Build history of the part. All positions in model axes, mm. Round coordinates to 2 decimals unless told otherwise and drop trailing zeros. Loops run counter-clockwise (first coordinate to the right, second up) from the corner with the lowest first, then second, coordinate; pieces in that order, holes last. Notation, with made-up numbers: (61, 48.25) - (78, 48.25) arc R14 ccw to (78, 70.25) - close; hole circle Ø2 at (75.25, 65.25). An arc over 180 degrees is marked (long way). Use a Markdown table: item, result.
Autodesk Inventor part; units mm, degrees
ref_plane "YZ Plane" through (0, 0, 0) normal (1, 0, 0) x (0, 1, 0)
ref_plane "XZ Plane" through (0, 0, 0) normal (0, 1, 0) x (-1, 0, 0)
ref_plane "XY Plane" through (0, 0, 0) normal (0, 0, 1) x (1, 0, 0)
sketch "Sketch1" plane through (0, 0, 0) normal (0, 0, 1) x (1, 0, 0)
  line L0 (-49.2977, 34.5359) -> (-22.38, 61.3045)
  line L1 (-47.8874, 33.1177) -> (-20.9698, 59.8864)
  line L2 (-49.2977, 34.5359) -> (-47.8874, 33.1177) construction
  circle A0 centre (-52.4729, 29.968) radius 5.563
  circle A1 centre (-52.4729, 29.968) radius 3.9984
  circle A2 centre (-17.7815, 64.4351) radius 5.563
  circle A3 centre (-17.7815, 64.4351) radius 3.9984
  line L3 (-13.9364, 68.4553) -> (0.7038, 78.9274)
  line L4 (-12.7631, 66.8356) -> (1.8771, 77.3077)
  line L5 (-57.711, 28.0946) -> (-68.2683, 22.3899)
  line L6 (-56.7093, 26.3625) -> (-67.2666, 20.6578)
  line L7 (-49.5894, 25.2106) -> (10.1162, -41.4966)
  circle A4 centre (14.4958, -44.9268) radius 5.563
  circle A5 centre (14.4958, -44.9268) radius 3.9984
  circle A6 centre (52.6405, -7.8239) radius 3.9984
  circle A7 centre (52.6405, -7.8239) radius 5.563
  line L8 (-48.0932, 26.5378) -> (11.6124, -40.1694)
  line L9 (-14.6001, 59.8716) -> (48.0505, -4.6808)
  line L10 (-13.1915, 61.292) -> (49.4591, -3.2604)
  line L11 (49.4227, -12.3618) -> (19.1106, -41.8201)
  line L12 (48.0258, -10.9306) -> (17.7136, -40.3888)
  line L13 (11.2885, -49.4721) -> (3.1929, -57.3557)
  line L14 (9.8883, -48.0441) -> (1.7927, -55.9277)
  line L15 (57.2511, -4.7111) -> (65.8331, 3.6764)
  line L16 (55.8523, -3.2817) -> (64.4343, 5.1058)
  line L17 (-39.0119, 41.9442) -> (29.6903, -28.7495)
  line L18 (-37.5936, 43.3546) -> (31.1246, -27.3556)
  line L19 (-55.5021, 34.6339) -> (-63.8979, 55.9393)
  line L20 (-53.6558, 35.4038) -> (-62.0516, 56.7092)
  line L21 (-23.223, 65.5915) -> (-56.073, 66.1322)
  line L22 (-23.2803, 63.5921) -> (-56.1303, 64.1329)
  circle A8 centre (-17.2221, 20.9576) radius 3.1804
  line L23 (13.0651, -39.5509) -> (-14.9644, 18.7175)
  line L24 (11.2563, -40.4044) -> (-16.7485, 17.8127)
  line L25 (-14.0533, 20.686) -> (47.9022, -4.9092)
  line L26 (-14.8421, 18.848) -> (47.1775, -6.7738)
  line L27 (-18.703, 58.9489) -> (-18.2564, 23.9652)
  line L28 (-16.7032, 58.9776) -> (-16.2565, 23.9879)
  line L29 (-47.4654, 27.5447) -> (-20.389, 20.6653)
  line L30 (-46.932, 29.4728) -> (-19.9371, 22.614)
  line L31 (0.7038, 78.9274) -> (1.8771, 77.3077)
  line L32 (-56.073, 66.1322) -> (-56.1303, 64.1329)
  line L33 (-62.0516, 56.7092) -> (-63.8979, 55.9393)
  line L34 (-68.2683, 22.3899) -> (-67.2666, 20.6578)
  line L35 (3.1929, -57.3557) -> (1.7927, -55.9277)
  line L36 (65.8331, 3.6764) -> (64.4343, 5.1058)
  point P0 (0, 0)
  point P1 (9.143, -43.4122)
  point P2 (-19.963, 60.8956)
  point P3 (18.6755, -41.2556)
  point P4 (19.8991, -43.603)
  point P5 (47.2964, -9.3692)
  point P6 (58.0343, -9.1855)
  point P7 (55.8444, -3.2761)
  point P8 (16.2732, -50.1982)
  point P9 (18.0227, -49.2289)
  point P10 (56.2951, -12.0181)
  point P11 (57.5423, -10.4544)
  point P12 (-20.321, 22.7115)
  point P13 (-20.9757, 59.8805)
  point P14 (-18.6091, 23.8197)
  point P15 (10.5981, -39.0362)
  point P16 (31.0842, -30.1838)
  point P17 (32.5185, -28.7899)
  point P18 (31.1246, -27.3556)
  point P19 (-13.0632, 18.1131)
  point P20 (-13.5186, 15.7119)
  point P21 (29.6903, -28.7495)
  point P22 (-20.0433, 22.4258)
  dimension "d49" = 6.3609
  dimension "d0" = 2
  dimension "d2" = 1
  dimension "d3" = 5.563
  dimension "d4" = 1.5646
  dimension "d6" = 1.5646
  dimension "d8" = 5.563
  dimension "d9" = 2
  dimension "d10" = 170.735
  dimension "d11" = 2
  dimension "d12" = 163.544
  dimension "d13" = 1.5646
  dimension "d17" = 7.9968
  dimension "d18" = 1.5646
  dimension "d19" = 7.9968
  dimension "d21" = 60.4275
  dimension "d22" = 66.8436
  dimension "d24" = 47.2075
  dimension "d25" = 2
  dimension "d26" = 2
  dimension "d27" = 81.433
  dimension "d28" = 93.011
  dimension "d29" = 53.2188
  dimension "d30" = 2
  dimension "d31" = 2
  dimension "d32" = 2
  dimension "d33" = 2
  dimension "d34" = 2
  dimension "d35" = 2
  dimension "d36" = 66.667
  dimension "d37" = 45.784
  dimension "d39" = 92.41
  dimension "d40" = 87.648
  dimension "d42" = 89.8
  dimension "d45" = 1
  dimension "d46" = 18
  dimension "d48" = 2
  dimension "d50" = 53.2132
  dimension "d51" = 27.126
  dimension "d52" = 44.9268
  dimension "d53" = 48.9027
  dimension "d54" = 29.968
  dimension "d55" = 20.9576
  dimension "d56" = 2
  dimension "d57" = 2
  dimension "d58" = 2
  dimension "d59" = 64.6596
  dimension "d60" = 67.0343
  dimension "d61" = 34.9897
  dimension "d62" = 27.8525
  dimension "d63" = 22.9
  dimension "d64" = 12
  dimension "d65" = 32.85
  dimension "d66" = 18
  dimension "d67" = 12
  dimension "d70" = 11.3
  dimension "d71" = 3.8451
  dimension "d72" = 5.4415
  dimension "d73" = 5.4358
  dimension "d74" = 5.2381
  dimension "d75" = 5.5409
  dimension "d76" = 5.4575
  dimension "d77" = 3.1128
  dimension "d78" = 2.6305
  dimension "d79" = 4.3021
extrude "Extrusion3" add sketch "Sketch1" against normal blind 1 contours L0 A2 L1 A0 | A0 | A2 | A0 L19 L33 L20 | L22 L32 L21 A2 | L1 L18 A8 L30 L17 | A2 L28 A8 L27 | L17 A8 L29 A0 L30 | A0 L6 L34 L5 | L3 L31 L4 A2 | A8 L18 | L18 A8 L17 | L17 A8 | A8 L25 A7 L26 L18 | L18 L26 A8 | A2 L10 A7 L9 | A8 L23 L17 | L17 L23 A4 L8 L24 A8 | L8 L24 A4 L7 A0 | L18 L12 L17 L23 A8 L26 | A7 | L8 A4 L24 | A4 | L12 A7 L11 A4 | A4 L13 L35 L14 | L16 L36 L15 A7
sketch "Sketch2" plane through (0, 0, 0) normal (0, 0, 1) x (1, 0, 0)
  circle A0 centre (52.6405, -7.8239) radius 3.9984
  circle A1 centre (52.6405, -7.8239) radius 3.9984
  circle A2 centre (14.4958, -44.9268) radius 3.9984
  circle A3 centre (14.4958, -44.9268) radius 3.9984
  circle A4 centre (-52.4729, 29.968) radius 3.9984
  circle A5 centre (-52.4729, 29.968) radius 3.9984
  circle A6 centre (-17.7815, 64.4351) radius 3.9984
  circle A7 centre (-17.7815, 64.4351) radius 3.9984
  point P0 (0, 0)
extrude "Extrusion2" add sketch "Sketch2" along normal blind 0.5 and the other way blind 1
equation "\"d6\" = d4"
equation "\"d13\" = d15"
equation "\"d18\" = d20"
properties part number "Grundform_Boden"
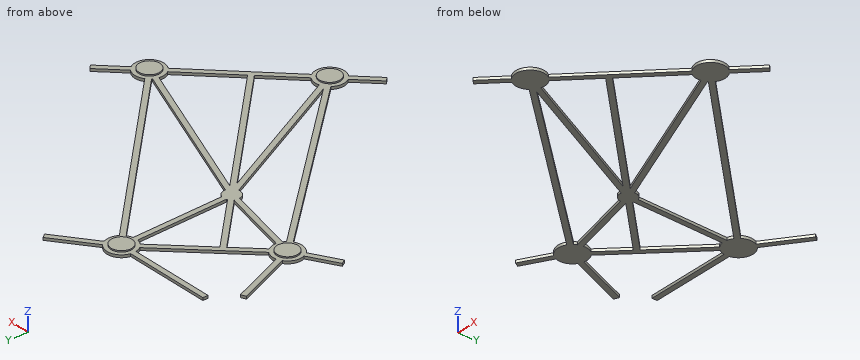
Q1. Cut at D-D, the plane z = 0.25. List the corners of the cut face in (x, y).
Results found:
| item | result |
|---|---|
| outline | circle Ø8 at (-52.47, 29.97); circle Ø8 at (-17.78, 64.44); circle Ø8 at (14.5, -44.93); circle Ø8 at (52.64, -7.82) |
Q2. Cut at C-C, the plane y = 10. List the corners of the cut face in (x, z).
Results found:
| item | result |
|---|---|
| outline | (-35.98, -1) - (-33.29, -1) - (-33.29, 0) - (-35.98, 0) - close; (-12.99, -1) - (-10.77, -1) - (-10.77, 0) - (-12.99, 0) - close; (-7.97, -1) - (-5.18, -1) - (-5.18, 0) - (-7.97, 0) - close; (6.58, -1) - (11.81, -1) - (11.81, 0) - (6.58, 0) - close; (33.8, -1) - (36.59, -1) - (36.59, 0) - (33.8, 0) - close |
Q3. Cut at B-B, the plane x = -29.5. List the corners of the cut face in (y, z), plus the area to 3 significant figures.
Results found:
| item | result |
|---|---|
| outline | (2.77, -1) - (5.76, -1) - (5.76, 0) - (2.77, 0) - close; (22.98, -1) - (25.04, -1) - (25.04, 0) - (22.98, 0) - close; (32.16, -1) - (35.03, -1) - (35.03, 0) - (32.16, 0) - close; (51.4, -1) - (54.22, -1) - (54.22, 0) - (51.4, 0) - close; (63.69, -1) - (65.69, -1) - (65.69, 0) - (63.69, 0) - close |
| area | 12.8 mm2 |
Q4. Probe line 1 (X direction, y = -11, z = -0.85); line 2 (X direction, y = 1.5, z = -0.85); line 3 (X direction, y = -26.5, z = -0.8). List the from-to ranges inside material, lowest first.
Results found:
| item | result |
|---|---|
| line 1 | x = -17.18 to -14.5, -2.89 to -0.67, 12.44 to 15.23, 47.95 to 57.21 |
| line 2 | x = -28.37 to -25.68, -8.9 to -6.68, 0.29 to 3.08, 27.15 to 32.39, 42.05 to 44.84, 60.74 to 63.61 |
| line 3 | x = -3.31 to -0.62, 4.57 to 6.79, 27.5 to 30.29, 32.01 to 34.87 |
Q5. Cut at A-A, the plane y = -25. List the corners of the cut face in (x, z).
Results found:
| item | result |
|---|---|
| outline | (-4.65, -1) - (-1.96, -1) - (-1.96, 0) - (-4.65, 0) - close; (3.85, -1) - (6.07, -1) - (6.07, 0) - (3.85, 0) - close; (26.05, -1) - (28.84, -1) - (28.84, 0) - (26.05, 0) - close; (33.55, -1) - (36.42, -1) - (36.42, 0) - (33.55, 0) - close |
Q6. Drop a flat-ended pin along its axis: pin 1 (10 mm diameter, centred on x = 26, y = -35.5, fed in from +Z). Give the stop position or say it passes through.
Results found:
| item | result |
|---|---|
| pin 1 | stops at z = 0 |
